Build history of the part. All positions in model axes, mm. A direction names the side the tool comes from. Give positions to 0.01 mm unless a question says otherwise; leave off trailing zeros. Loops run counter-clockwise (first coordinate to the right, second up) from the corner with the lowest first, then second, coordinate; pieces in that order, holes last.
1) Band-saw the part on B-B on y = -1.75. List the corners of the cut face in (x, z), then the cut area to 3 significant figures.
2) Band-saw the part on C-C on z = 4.25. List the corners of the cut face in (x, y), then the cut area to 3 significant figures.
3) Band-saw the part on A-A on x = -20.5. List the corners of the cut face in (y, z).
4) Wall check: line 1 (Y direction, x = -22, z = 5.75); line 2 (Z direction, x = 3, y = -1.5); line 3 (X direction, y = 3, z = 5). Give the ranges that are in metal, low to high.
5) Flat gauge pins, fed straight in: P1, Ø4, axis at y = 2.5, z = 6, coming from the +X side; P2, Ø3, axis at y = -0.5, z = 2, coming from the -X side; P3, Ø1.6, axis at y = 0, z = 4, coming from the +X side. Where does each tip first touch, or does it go through?
6) 3-axis set-ups, long thin cutter, end or side, ignore diameter. For faces 1 (the flat face through (0.942, -1, 5)), 2 (the flat face through (-7, -1, 0)), 3 (the flat face through (-22, 1.889, 5)): which of +Z, -Z, +X, -X, +Y, -Y reach the whole face in a straight line?
7) Band-saw the part on D-D on y = 3. List the corners of the cut face in (x, z).
8) Two-plate mould, pull along Y, no slides. Class faces 4 (the flat face through (-12, 4.139, 5)), 5 (the cylindrical face through (5.23, -2.24, 8.86)), 6 (the flat face through (-19.058, -1, 5)), 7 (the flat face through (4, -1, 2.25)): +Y half, -Y half, draft (parallel to the pull), parting line (faces both ways), or undercut.
```python
from build123d import *

# Parameters (mm, degrees)
SKETCH1_W            = 30
SKETCH1_H            = 10
BOSS_EXTRUDE1_DEPTH  = 10
SKETCH2_R            = 5
BOSS_EXTRUDE2_DEPTH  = 2.25
BOSS_EXTRUDE4_DEPTH  = 2.25
MIRROR4_COPY_1_DEPTH = 2.25
MIRROR4_COPY_2_DEPTH = 2.25
SKETCH4_R            = 1.9
CUT_EXTRUDE1_DEPTH   = 13.25
SKETCH5_R            = 1.55
CUT_EXTRUDE2_DEPTH   = 13.25
SKETCH6_W            = 5
SKETCH6_H            = 5.5
CUT_EXTRUDE3_DEPTH   = 13.25
SKETCH7_W            = 5
SKETCH7_H            = 5.5
CUT_EXTRUDE4_DEPTH   = 13.25


with BuildPart() as part:
    # Sketch1 → Boss-Extrude1 (new body)
    with BuildSketch(Plane.XY):
        with Locations((-9.058394161, -0.861313869)):
            Rectangle(SKETCH1_W, SKETCH1_H)
    extrude(amount=BOSS_EXTRUDE1_DEPTH)

    # Sketch2 → Boss-Extrude2 (add)
    with BuildSketch(Plane.XY.offset(10)):
        with Locations((5.941605839, -0.861313869)):
            Circle(SKETCH2_R)
    boss_extrude2 = extrude(amount=-BOSS_EXTRUDE2_DEPTH)

    # Sketch3 → Boss-Extrude4 (add)
    with BuildSketch(Plane(origin=(0, 4.138686131, 0), x_dir=(1, 0, 0), z_dir=(0, 1, 0))):
        with BuildLine():
            Line((-24.058394161, -10), (-24.058394161, -5))
            Line((-24.058394161, -5), (-29.058394161, -5))
            ThreePointArc((-29.058394161, -5), (-27.593928067, -8.535533906), (-24.058394161, -10))
        make_face()
    boss_extrude4 = extrude(amount=-BOSS_EXTRUDE4_DEPTH)

    # Mirror1: Boss-Extrude2, Boss-Extrude4 across plane
    add(boss_extrude2.mirror(Plane(origin=(0, 0, 5), x_dir=(1, 0, 0), z_dir=(0, 0, -1))))
    add(boss_extrude4.mirror(Plane(origin=(0, 0, 5), x_dir=(1, 0, 0), z_dir=(0, 0, -1))))

    # Mirror3: Boss-Extrude4 across plane
    add(boss_extrude4.mirror(Plane.ZX.offset(-0.861313869)))

    # Mirror4 copy 1 sketch → Mirror4 copy 1 (add)
    with BuildSketch(Plane(origin=(0, -5.861313869, 10), x_dir=(1, 0, 0), z_dir=(0, -1, 0))):
        with BuildLine():
            Line((-24.058394161, -10), (-24.058394161, -5))
            Line((-24.058394161, -5), (-29.058394161, -5))
            ThreePointArc((-29.058394161, -5), (-27.593928067, -8.535533906), (-24.058394161, -10))
        make_face()
    extrude(amount=-MIRROR4_COPY_1_DEPTH)

    # Mirror4 copy 2 sketch → Mirror4 copy 2 (add)
    with BuildSketch(Plane(origin=(0, 4.138686131, 10), x_dir=(1, 0, 0), z_dir=(0, 1, 0))):
        with BuildLine():
            Line((-24.058394161, 10), (-24.058394161, 5))
            Line((-24.058394161, 5), (-29.058394161, 5))
            ThreePointArc((-29.058394161, 5), (-27.593928067, 8.535533906), (-24.058394161, 10))
        make_face()
    extrude(amount=-MIRROR4_COPY_2_DEPTH)

    # Sketch4 → Cut-Extrude1 (cut)
    with BuildSketch(Plane(origin=(0, 4.138686131, 0), x_dir=(1, 0, 0), z_dir=(0, 1, 0))):
        with Locations(Location((-24.058394161, -5, 0), (0, 0, 270))):  # turned: the seam where the file's is
            Circle(SKETCH4_R)
    extrude(amount=-CUT_EXTRUDE1_DEPTH, mode=Mode.SUBTRACT)

    # Sketch5 → Cut-Extrude2 (cut)
    with BuildSketch(Plane(origin=(0, 0, 0), x_dir=(-1, 0, 0), z_dir=(0, 0, -1))):
        with Locations((-5.941605839, -0.861313869)):
            Circle(SKETCH5_R)
    extrude(amount=-CUT_EXTRUDE2_DEPTH, mode=Mode.SUBTRACT)

    # Sketch6 → Cut-Extrude3 (cut)
    with BuildSketch(Plane(origin=(0, 4.138686131, 0), x_dir=(1, 0, 0), z_dir=(0, 1, 0))):
        with Locations((3.441605839, -5)):
            Rectangle(SKETCH6_W, SKETCH6_H)
    extrude(amount=-CUT_EXTRUDE3_DEPTH, mode=Mode.SUBTRACT)

    # Sketch7 → Cut-Extrude4 (cut)
    with BuildSketch(Plane.XY.offset(10)):
        with Locations((-21.558394161, -0.861313869)):
            Rectangle(SKETCH7_W, SKETCH7_H)
    extrude(amount=-CUT_EXTRUDE4_DEPTH, mode=Mode.SUBTRACT)


solid = part.part
```
Findings below:
1. outline: (-19.06, 0) - (4.67, 0) - (4.67, 2.25) - (0.94, 2.25) - (0.94, 7.75) - (4.67, 7.75) - (4.67, 10) - (-19.06, 10) - close; (7.21, 0) - (10.86, 0) - (10.86, 2.25) - (7.21, 2.25) - close; (7.21, 7.75) - (10.86, 7.75) - (10.86, 10) - (7.21, 10) - close
1. area: 233 mm2
2. outline: (-29, -5.86) - (-25.8, -5.86) - (-25.8, -3.61) - (-29, -3.61) - close; (-29, 1.89) - (-25.8, 1.89) - (-25.8, 4.14) - (-29, 4.14) - close; (-22.31, -5.86) - (0.94, -5.86) - (0.94, 4.14) - (-22.31, 4.14) - (-22.31, 1.89) - (-19.06, 1.89) - (-19.06, -3.61) - (-22.31, -3.61) - close
2. area: 229 mm2
3. outline: (-5.86, 0) - (-3.61, 0) - (-3.61, 10) - (-5.86, 10) - close; (1.89, 0) - (4.14, 0) - (4.14, 10) - (1.89, 10) - close
4. line 1: y = -5.86 to -3.61, 1.89 to 4.14
4. line 2: z = 0 to 2.25, 7.75 to 10
4. line 3: x = -29.06 to -25.96, -22.16 to 0.94
5. P1: stops at x = 10.33
5. P2: stops at x = -19.06
5. P3: stops at x = 0.94
6. face 1: +X, +Y, -Y
6. face 2: -Z, +X, -X, +Y, -Y
6. face 3: +Z, -Z, -X
7. outline: (-24.06, 0) - (9.12, 0) - (9.12, 2.25) - (0.94, 2.25) - (0.94, 7.75) - (9.12, 7.75) - (9.12, 10) - (-24.06, 10) arc R5 ccw to start; hole circle Ø3.8 at (-24.06, 5)
8. face 4: +Y half
8. face 5: undercut
8. face 6: undercut
8. face 7: draft
